from build123d import *

# Parameters (mm, degrees)
PAD_DEPTH       = 8
POCKET_DEPTH    = 6.5
SKETCH_R        = 1.5
POCKET001_DEPTH = 8.001
FILLET_R        = 0.5


with BuildPart() as part:
    # Sketch004 (on XY_Plane of Origin) → Pad (new body)
    with BuildSketch(Plane.XY):
        with BuildLine():
            ThreePointArc((0.198755, -2.434603), (1.728484, -4.835416), (3.775997, -6.813208))
            ThreePointArc((3.775997, -6.813208), (4.37324, -7.125), (5.040127, -7.220785))
            Line((5.040127, -7.220785), (13.436073, -6.997526))
            ThreePointArc((13.436073, -6.997526), (18.265103, -4.883518), (20.25, 0))
            Line((0, 0), (20.25, 0))
            Line((0, 0), (0, -1.565397))
            ThreePointArc((0, -1.565397), (0.050322, -2.011217), (0.198755, -2.434603))
        make_face()
    pad = extrude(amount=PAD_DEPTH)

    # Mirrored: Pad across Sketch004 H_Axis
    add(pad.mirror(Plane.ZX))

    # Sketch005 (on Face5 of Mirrored) → Pocket (cut)
    with BuildSketch(Plane.XY.offset(8)):
        with BuildLine():
            Line((17.291658, -4.125), (20.291658, -4.125))
            Line((20.291658, -4.125), (20.291658, 0))
            Line((20.291658, 0), (6.208342, 0))
            Line((6.208342, -4.125), (6.208342, 0))
            Line((9.208342, -4.125), (6.208342, -4.125))
            ThreePointArc((9.208342, -4.125), (13.25, -5.775), (17.291658, -4.125))
        make_face()
    pocket = extrude(amount=-POCKET_DEPTH, mode=Mode.SUBTRACT)

    # Mirrored001: Pocket across Sketch005 H_Axis
    add(pocket.mirror(Plane(origin=(0, 0, 8), x_dir=(0, 0, 1), z_dir=(0, 1, 0))), mode=Mode.SUBTRACT)

    # Sketch (on XY_Plane of Origin) → Pocket001 (cut, through all)
    with BuildSketch(Plane.XY):
        with Locations((13.25, 0)):
            Circle(SKETCH_R)
    extrude(amount=POCKET001_DEPTH, mode=Mode.SUBTRACT)

    # Fillet
    fillet_edges = [part.edges().sort_by_distance(p)[0] for p in [
        (6.208342, 4.125, 4.75),
        (6.208342, -4.125, 4.75),
    ]]
    fillet(fillet_edges, radius=FILLET_R)


solid = part.part
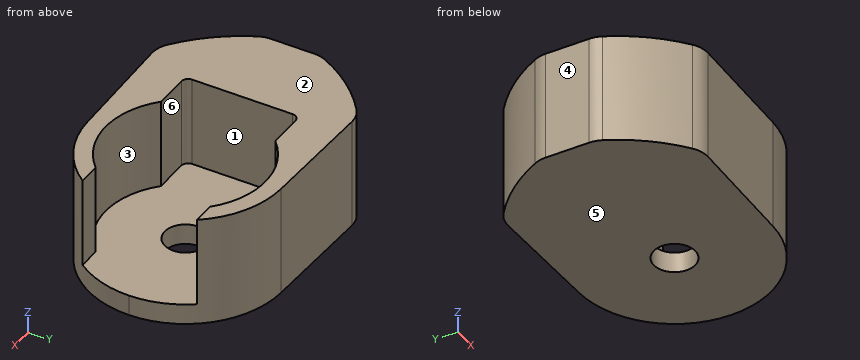
Check sheet for the modelled part. Datum: model origin and axes. Units: mm. Face numbers are marked on the shaded views. A direction names the side the tool comes from. Round coordinates to 2 decimals unless told otherwise and drop trailing zeros. Order: outer loops, then holes, each group sorted by start corner. A loop starts at its lowest first (then second) coordinate and runs counter-clockwise, first axis right, second up. Notation, with made-up numbers: M 1,88 L 25,88 A28 ccw 25,111 Z; hole C 30,28.25 d10. An arc over 180 degrees is marked long. One line per item, written item: value. Start each with the question number.
1. Scan lines: line 1 along Y through (x, z) = (13.25, 0.3); line 2 along X through (y, z) = (0, 1.15); line 3 along Z through (x, y) = (16, 0.5). Record each from-to range of solid material in increasing order.
2. Section check B-B on x = 12.5. Enter the section's corners in (y, z).
3. Section check A-A on z = 0.5. Enter the section's corners in (x, y), and give its area (3 significant figures).
4. Section check D-D on y = -1.25. Enter the section's corners in (x, z), and give its area (3 significant figures).
5. Access from +Z, -Z, +X, -X, +Y, -Y to the whole of each face (thin tool, end or side, straight path). Record for the marked faces 5 and 6.
6. Release check for a two-part mould opening along X. For the marked faces 1, 2, 3 and 4 record: released by +X, released by -X, zero draft, split by the parting line, or undercut.
7. Gauge pin test, flat ends, axial feed: P1, Ø2, axis at x = 16, z = 4.5, coming from the +Y side; P2, Ø1.8, axis at x = 17.5, z = 5.5, coming from the +Y side; P3, Ø0.8, axis at x = 8, z = 6, coming from the -Y side. Record the tip position at first contact, or that the pin passes through.
Results found:
1. line 1: -7 to -1.5, 1.5 to 7
1. line 2: 0 to 11.75, 14.75 to 20.25
1. line 3: 0 to 1.5
2. outline: M -7.02,0 L -1.3,0 L -1.3,1.5 L -5.73,1.5 L -5.73,8 L -7.02,8 Z; M 1.3,0 L 7.02,0 L 7.02,8 L 5.73,8 L 5.73,1.5 L 1.3,1.5 Z
3. outline: M 0,-1.57 A2 ccw 0.2,-2.43 A12.12 ccw 3.78,-6.81 A2 ccw 5.04,-7.22 L 13.44,-7 A7 ccw 20.25,0 A7 ccw 13.44,7 L 5.04,7.22 A2 ccw 3.78,6.81 A12.12 ccw 0.2,2.43 A2 ccw 0,1.57 Z; hole C 13.25,0 d3
3. area: 241 mm^2
4. outline: M 0,0 L 12.42,0 L 12.42,1.5 L 6.21,1.5 L 6.21,8 L 0,8 Z; M 14.08,0 L 20.14,0 L 20.14,1.5 L 14.08,1.5 Z
4. area: 68.1 mm^2
5. face 5: -Z, +X, -X, +Y, -Y
5. face 6: +Z, +X
6. face 1: released by +X
6. face 2: zero draft
6. face 3: undercut
6. face 4: released by -X
7. P1: y = 6.78
7. P2: y = 6.15
7. P3: y = -7.15
